```python
from build123d import *

# Parameters (mm, degrees)
F0_R     = 112.5
F1_DEPTH = 10
F2_R     = 30
F3_DEPTH = 10
F5_D     = 12.5


with BuildPart() as f1:
    # F0 (on Top) → F1 (new body)
    with BuildSketch(Plane.XY):
        Circle(F0_R)
    extrude(amount=F1_DEPTH)

    # F2 (on face) → F3 (cut, through all)
    with BuildSketch(Plane.XY.offset(10)):
        Circle(F2_R)
    extrude(amount=-F3_DEPTH, mode=Mode.SUBTRACT)

    # F5 (through all)
    with Locations(Plane.XY.offset(10)):
        with Locations((85, 0), (68.766445, -49.961746), (68.766445, 49.961746), (26.266445, 80.839804), (-26.266445, 80.839804), (-68.766445, 49.961746), (-85, 0), (-68.766445, -49.961746), (-26.266445, -80.839804), (26.266445, -80.839804)):
            Hole(F5_D / 2)


solid = f1.part
```
Model file for the job. Use its own axes, mm. Round coordinates to 2 decimals unless told otherwise and drop trailing zeros. Order: outer loops, then holes, each group sorted by start corner. A loop starts at its lowest first (then second) coordinate and runs counter-clockwise, first axis right, second up. Notation, with made-up numbers: M 43,58.5 L 55,58.5 A19 cw 55,72.5 Z; hole C -32,45.5 d2. An arc over 180 degrees is marked long. Use CSV: the item, a comma, the result in double quotes.
Item 1: Pin check, flat tips, straight feed: pin 1 (4 mm diameter, centred on x = 64, z = 7, fed in from +Y); pin 2 (2 mm diameter, centred on y = -43.5, z = 7.5, fed in from +X); pin 3 (2 mm diameter, centred on y = -81, z = 6.5, fed in from +X). Stop position of each tip, or through.
Worked answers:
pin 1,"y = 93.87"
pin 2,"x = 104.16"
pin 3,"x = 79.1"
Item 2: Pull direction Y, two halves, no side cores. Call faces 1 (the face through (-112.39, 4.95, 4.93)), 2 (the face through (23, -23, 10)), 3 (the face through (27.08, 87.037, 4.93)), 4 (the face through (-90.96, 1.88, 4.93)): released by +Y, released by -Y, zero draft, split by the parting line, or undercut.
Worked answers:
face 1,"split by the parting line"
face 2,"zero draft"
face 3,"undercut"
face 4,"undercut"
Item 3: Saw through at A-A (y = 0). List the corners of the cut face in (x, z), plus the area to 3 significant figures.
Worked answers:
outline,"M -112.5,0 L -91.25,0 L -91.25,10 L -112.5,10 Z; M -78.75,0 L -30,0 L -30,10 L -78.75,10 Z; M 30,0 L 78.75,0 L 78.75,10 L 30,10 Z; M 91.25,0 L 112.5,0 L 112.5,10 L 91.25,10 Z"
area,"1,400 mm²"
Item 4: Probe probe 1 along X at (y, z) = (-49.5, 3.5); probe 2 along X at (y, z) = (78, 4.5); probe 3 along Y at (x, z) = (-73.5, 2.75). List the from-to ranges inside material, lowest first.
Worked answers:
probe 1,"-101.02 to -75, -62.53 to 62.53, 75 to 101.02"
probe 2,"-81.07 to -31.83, -20.7 to 20.7, 31.83 to 81.07"
probe 3,"-85.17 to -54.04, -45.88 to 45.88, 54.04 to 85.17"
Item 5: Saw through at B-B (x = 0). List the corners of the cut face in (y, z).
Worked answers:
outline,"M -112.5,0 L -30,0 L -30,10 L -112.5,10 Z; M 30,0 L 112.5,0 L 112.5,10 L 30,10 Z"
Item 6: Saw through at D-D (x = -85). List the corners of the cut face in (y, z), plus the area to 3 significant figures.
Worked answers:
outline,"M -73.7,0 L -6.25,0 L -6.25,10 L -73.7,10 Z; M 6.25,0 L 73.7,0 L 73.7,10 L 6.25,10 Z"
area,"1,350 mm²"
Item 7: Saw through at C-C (z = 8). State how many separate pieces and enclosed holes the cut face has, plus the area to 3 significant figures.
Worked answers:
separate pieces,"1"
enclosed holes,"11"
area,"35,700 mm²"
